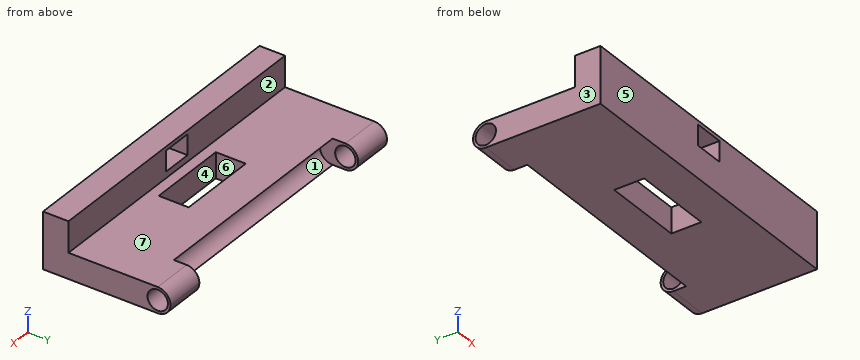
```python
from build123d import *

# Parameters (mm, degrees)
F0_W      = 76.2
F0_H      = 25.4
F2_DEPTH  = 6.35
F1_W      = 20.0991295278
F1_H      = 7.4727535248
F3_DEPTH  = 6.35
F4_W      = 10.16
F4_H      = 6.35
F5_DEPTH  = 19.05
F6_R      = 2.54
F7_DEPTH  = 76.2
F8_DEPTH  = 76.2
F10_DEPTH = 27.94
F11_W     = 76.2
F11_H     = 6.35
F12_DEPTH = 13.97
F13_W     = 7.62
F13_H     = 5.08
F14_DEPTH = 25.4
F15_DEPTH = 190.5


with BuildPart() as f2:
    # F0 (on Top) → F2 (new body)
    with BuildSketch(Plane.XY):
        Rectangle(F0_W, F0_H)
    extrude(amount=F2_DEPTH)

    # F1 (on Top) → F3 (cut)
    with BuildSketch(Plane.XY):
        Rectangle(F1_W, F1_H)
    extrude(amount=F3_DEPTH, mode=Mode.SUBTRACT)

    # F4 (on Front) → F5 (join)
    with BuildSketch(Plane.XZ):
        with Locations((33.02, 3.175)):
            Rectangle(F4_W, F4_H)
        with Locations((-33.02, 3.175)):
            Rectangle(F4_W, F4_H)
    extrude(amount=-F5_DEPTH)

    # F6 (on face) → F7 (cut)
    with BuildSketch(Plane(origin=(-38.1, 0, 0), x_dir=(0, -1, 0), z_dir=(-1, 0, 0))):
        with Locations((-15.875, 3.175)):
            Circle(F6_R)
    extrude(amount=-F7_DEPTH, mode=Mode.SUBTRACT)

    # F6 (on face) → F8 (cut)
    with BuildSketch(Plane(origin=(-38.1, 0, 0), x_dir=(0, -1, 0), z_dir=(-1, 0, 0))):
        with BuildLine():
            Line((-19.05, 0), (-15.875, 0))
            ThreePointArc((-15.875, 0), (-18.1200640303, 0.9299359697), (-19.05, 3.175))
            Line((-19.05, 3.175), (-19.05, 0))
        make_face()
        with BuildLine():
            ThreePointArc((-19.05, 3.175), (-18.1200640229, 5.4200640376), (-15.8749999792, 6.35))
            Line((-15.8749999792, 6.35), (-19.05, 6.35))
            Line((-19.05, 6.35), (-19.05, 3.175))
        make_face()
    extrude(amount=-F8_DEPTH, mode=Mode.SUBTRACT)

    # F9 (on Right) → F10 (cut, symmetric)
    with BuildSketch(Plane.YZ):
        with BuildLine():
            ThreePointArc((12.7, 6.35), (9.525, 3.175), (12.7, 0))
            Line((12.7, 0), (12.7, 6.35))
        make_face()
    extrude(amount=F10_DEPTH, both=True, mode=Mode.SUBTRACT)

    # F11 (on Top) → F12 (join)
    with BuildSketch(Plane.XY):
        with Locations((0, -9.525)):
            Rectangle(F11_W, F11_H)
    extrude(amount=F12_DEPTH)

    # F13 (on face) → F14 (join)
    with BuildSketch(Plane.XZ.offset(12.7)):
        with Locations((0, 10.4701574892)):
            Rectangle(F13_W, F13_H)
    extrude(amount=F14_DEPTH)

    # F15 (cut, symmetric): a face of the model
    f15_faces = [f2.faces().sort_by_distance(p)[0] for p in [
        (0, -38.1, 10.4701574892),
    ]]
    extrude(f15_faces, amount=F15_DEPTH, both=True, mode=Mode.SUBTRACT)


solid = f2.part
```
Input: part model. Units: mm. Frame: model coordinates. Face numbers are marked on the shaded views. A direction names the side the tool comes from. Round coordinates to 2 decimals unless told otherwise and drop trailing zeros. Loops run counter-clockwise (first coordinate to the right, second up) from the corner with the lowest first, then second, coordinate; pieces in that order, holes last. Notation, with made-up numbers: (-0.75, -2.75) -> (15.25, -2.75) arc R30 ccw to (15.25, 22.25) -> close; hole circle Ø9 at (69.5, 15). An arc over 180 degrees is marked (long way). Use one line per item in the form item = value. Start each with the question number.
Item 1: Section query C-C on x = -12. Return the cut outline in (y, z) (3 decimals).
Item 2: Set-up query: the marked faces 1, 2, 3 and 4. Return all of +Z, -Z, +X, -X, +Y, -Y with unobstructed straight access to the full face (end or side cutting, diameter ignored); none if empty.
Item 3: Section query B-B on x = 30. Return the cut outline in (y, z) (3 decimals), then the cut area to 3 significant figures.
Item 4: Section query A-A on z = 11.5. Return the cut outline in (x, y), then the cut area to 3 significant figures.
Item 5: Material intervals for L1, parallel to X at y = 11, z = 3.75; L2, parallel to Z at x = 10.5, y = 7; L3, parallel to Y at x = -35, z = 11.25, sorted ascending. Write a range as from..to.
Item 6: Mould query, pull axis Y, two halves, no side actions, for the marked faces 5, 6 and 7. Classes: pulls with the +Y half, pulls with the -Y half, needs draft (parallel to the pull), parting line crosses it, or undercut.
Item 7: Contact query for flat-ended pins moving along their axis: pin 1 Ø18 at (x, y) = (16.5, 5.5) entering from +Z; pin 2 Ø1.9 at (x, z) = (3, 4) entering from +Y; pin 3 Ø4 at (x, z) = (3, 8.5) entering from +Y. Output: stop coordinate, or through.
Item 8: Section query D-D on y = 6. Return the cut outline in (x, z).
Ans:
q1.outline = (-12.7, 0) -> (12.7, 0) arc R3.175 cw to (12.7, 6.35) -> (-6.35, 6.35) -> (-6.35, 13.97) -> (-12.7, 13.97) -> close
q2.face_1 = +Y
q2.face_2 = +Z, +X, -X, +Y
q2.face_3 = +Z, -Z, -X, +Y, -Y
q2.face_4 = +Z, -Z
q3.outline = (-12.7, 0) -> (15.875, 0) arc R3.175 ccw to (15.875, 6.35) -> (-6.35, 6.35) -> (-6.35, 13.97) -> (-12.7, 13.97) -> close; hole circle Ø5.08 at (15.875, 3.175)
q3.area = 225 mm^2
q4.outline = (-38.1, -12.7) -> (-3.81, -12.7) -> (-3.81, -6.35) -> (-38.1, -6.35) -> close; (3.81, -12.7) -> (38.1, -12.7) -> (38.1, -6.35) -> (3.81, -6.35) -> close
q4.area = 435 mm^2
q5.L1 = -38.1..-27.94, 27.94..38.1
q5.L2 = 0..6.35
q5.L3 = -12.7..-6.35
q6.face_5 = pulls with the -Y half
q6.face_6 = undercut
q6.face_7 = needs draft
q7.pin_1 = 6.35
q7.pin_2 = 10.07
q7.pin_3 = -6.35
q8.outline = (-38.1, 0) -> (38.1, 0) -> (38.1, 6.35) -> (-38.1, 6.35) -> close
